The model under review builds one solid part; all positions refer to its coordinate system, in mm. A direction names the side the tool comes from. Coordinates: 2 decimals unless noted, no trailing zeros. Write each loop counter-clockwise with the first axis right and the second up, starting at its lowest first coordinate (ties: lowest second). Pieces come first, ordered by that corner, then holes.
1) For P1, Ø6, axis at y = 14, z = -95.5, coming from the -X side; P2, Ø12, axis at y = -26, z = -44.5, coming from the -X side; P3, Ø2, axis at x = 84, y = -4, coming from the -Z side, all flat-tipped, find the tip position at first contact; note any pin that passes through.
2) Machinability: for faces 1 (the cylindrical face through (186.385, 9.011, -99.3)), 2 (the flat face through (71, -40, 0)), 3 (the flat face through (164, -1, 50)), 4 (the flat face through (51, 1, -7.5)), which of the approach directions +Z, -Z, +X, -X, +Y, -Y give a long, thin tool a straight path to every point of the face, cutting with its end or side? Answer none if there is none.
3) For line 1 (Z direction, x = 185, y = -37); line 2 (X direction, y = -17, z = 25); line 3 (Z direction, x = 265, y = 39), list the stretches that pass through material, from the lowest coordinate up.
4) Add section C-C, the plane z = -40. State the section outline as (x, y) points, then the cut area to 3 significant figures.
5) Add section A-A, the plane y = 0. State the section outline as (x, z) points.
6) Add section D-D, the plane x = 107. State the section outline as (y, z) points, then the cut area to 3 significant figures.
7) Add section B-B, the plane x = 215. State the section outline as (y, z) points, then the cut area to 3 significant figures.
from build123d import *

# Parameters (mm, degrees)
BOSS_EXTRUDE1_DEPTH = 7.5
SKETCH3_W           = 100
SKETCH3_H           = 130
BOSS_EXTRUDE2_DEPTH = 150
SKETCH4_R           = 30
BOSS_EXTRUDE3_DEPTH = 100
SKETCH5_R           = 50
BOSS_EXTRUDE4_DEPTH = 50
SKETCH6_R           = 25
BOSS_EXTRUDE5_DEPTH = 100


with BuildPart() as part:
    # Sketch1 → Boss-Extrude1 (new body, symmetric)
    with BuildSketch(Plane.XY):
        with BuildLine():
            Line((0, 40), (140, 40))
            Line((140, 40), (140, -40))
            Line((140, -40), (0, -40))
            ThreePointArc((0, -40), (-40, 0), (0, 40))
        make_face()
    extrude(amount=BOSS_EXTRUDE1_DEPTH, both=True)

    # Sketch3 → Boss-Extrude2 (add)
    with BuildSketch(Plane(origin=(140, 0, 0), x_dir=(0, 0, -1), z_dir=(1, 0, 0))):
        Rectangle(SKETCH3_W, SKETCH3_H)
    extrude(amount=BOSS_EXTRUDE2_DEPTH)

    # Sketch4 → Boss-Extrude3 (add)
    with BuildSketch(Plane(origin=(0, 0, -50), x_dir=(-1, 0, 0), z_dir=(0, 0, -1))):
        with Locations((-215, 0)):
            Circle(SKETCH4_R)
    extrude(amount=BOSS_EXTRUDE3_DEPTH)

    # Sketch5 → Boss-Extrude4 (add)
    with BuildSketch(Plane.XY.offset(50)):
        with Locations((215, 0)):
            Circle(SKETCH5_R)
    extrude(amount=BOSS_EXTRUDE4_DEPTH)

    # Sketch6 → Boss-Extrude5 (add)
    with BuildSketch(Plane.XY.offset(100)):
        with Locations((215, 0)):
            Circle(SKETCH6_R)
    extrude(amount=BOSS_EXTRUDE5_DEPTH)


solid = part.part
Geometry results:
1. P1: stops at x = 187.09
1. P2: stops at x = 140
1. P3: stops at z = -7.5
2. face 1: -Z
2. face 2: +Z, -Z, -X, -Y
2. face 3: +Z
2. face 4: -Z, -X, +Y, -Y
3. line 1: z = -50 to 100
3. line 2: x = 140 to 290
3. line 3: z = -50 to 50
4. outline: (140, -65) - (290, -65) - (290, 65) - (140, 65) - close
4. area: 19,500 mm2
5. outline: (-40, -7.5) - (140, -7.5) - (140, -50) - (185, -50) - (185, -150) - (245, -150) - (245, -50) - (290, -50) - (290, 50) - (265, 50) - (265, 100) - (240, 100) - (240, 200) - (190, 200) - (190, 100) - (165, 100) - (165, 50) - (140, 50) - (140, 7.5) - (-40, 7.5) - close
6. outline: (-40, -7.5) - (40, -7.5) - (40, 7.5) - (-40, 7.5) - close
6. area: 1,200 mm2
7. outline: (-65, -50) - (-30, -50) - (-30, -150) - (30, -150) - (30, -50) - (65, -50) - (65, 50) - (50, 50) - (50, 100) - (25, 100) - (25, 200) - (-25, 200) - (-25, 100) - (-50, 100) - (-50, 50) - (-65, 50) - close
7. area: 29,000 mm2
